Build history of the part. All positions in model axes, mm. A direction names the side the tool comes from. Give positions to 0.01 mm unless a question says otherwise; leave off trailing zeros. Loops run counter-clockwise (first coordinate to the right, second up) from the corner with the lowest first, then second, coordinate; pieces in that order, holes last. Notation, with made-up numbers: M -19,46 L -15,46 A28 ccw -15,69 Z; hole C 15,-31.5 d1. An arc over 180 degrees is marked long. Answer as a JSON object with one key per item and string values. Group by question number.
1. Drill centre lines: line 1 along Y through (x, z) = (35, 3); line 2 along Z through (x, y) = (0, -4.5); line 3 along Z through (x, y) = (-44, -4). Where is each one in solid material? Low to high. Write a range as [from, to].
2. Slice it at C-C (z = 27.5). List the corners of the cut face in (x, y), then the cut area to 3 significant figures.
3. Slice it at A-A (x = -35). List the corners of the cut face in (y, z).
4. Drop flat-ended pins along their axis: pin 1 Ø1.5 at (y, z) = (-15, 49) entering from +X; pin 2 Ø11 at (y, z) = (-7.5, 32.5) entering from -X; pin 3 Ø7 at (y, z) = (-7, 33.5) entering from +X. Give the stop position or say it passes through.
5. 3-axis set-ups, long thin cutter, end or side, ignore diameter. For faces 1 (the face through (-20, -10, 29)), 2 (the face through (-1, 0, 0)), 3 (the face through (0, 0, 33)): which of +Z, -Z, +X, -X, +Y, -Y reach the whole face in a straight line?
6. Slice it at B-B (y = -4). List the corners of the cut face in (x, z), then the cut area to 3 significant figures.
7. Slice it at D-D (z = 8). List the corners of the cut face in (x, y), then the cut area to 3 significant figures.
8. Mould opens along Y. For faces 4 (the face through (-31.38, -19.14, 14.1)), 5 (the face through (-40, 10, 7)), 6 (the face through (1, 20, 6)) say: released by +Y, released by -Y, zero draft, split by the parting line, or undercut.
from build123d import *

# Parameters (mm, degrees)
F0_R     = 5
F0_W     = 40
F0_H     = 40
F1_DEPTH = 15
F2_R     = 5
F3_DEPTH = 20
F4_R     = 3


with BuildPart() as f1:
    # F0 (on Top) → F1 (new body)
    with BuildSketch(Plane.XY):
        with BuildLine():
            Line((-40, -20), (-20.3233100474, -20))
            Line((-20.3233100474, -20), (-20.3233100474, 20))
            Line((-20.3233100474, 20), (-40, 20))
            ThreePointArc((-40, 20), (-47.0710678119, 17.0710678119), (-50, 10))
            Line((-50, 10), (-50, -10))
            ThreePointArc((-50, -10), (-47.0710678119, -17.0710678119), (-40, -20))
        make_face()
        with Locations((-35, 10)):
            Circle(F0_R, mode=Mode.SUBTRACT)
        with Locations((-0.3233100474, 0)):
            Rectangle(F0_W, F0_H)
        with BuildLine():
            Line((19.6766899526, -20), (40, -20))
            ThreePointArc((40, -20), (47.0710678119, -17.0710678119), (50, -10))
            Line((50, -10), (50, 10))
            ThreePointArc((50, 10), (47.0710678119, 17.0710678119), (40, 20))
            Line((40, 20), (19.6766899526, 20))
            Line((19.6766899526, 20), (19.6766899526, -20))
        make_face()
        with Locations((35, 10)):
            Circle(F0_R, mode=Mode.SUBTRACT)
    extrude(amount=F1_DEPTH)

    # F2 (on face) → F3 (join)
    with BuildSketch(Plane.XZ.offset(20)):
        with BuildLine():
            ThreePointArc((20, 40), (0, 60), (-20, 40))
            Line((-20, 40), (-20, 15))
            Line((-20, 15), (20, 15))
            Line((20, 15), (20, 40))
        make_face()
        with Locations((0, 40)):
            Circle(F2_R, mode=Mode.SUBTRACT)
    extrude(amount=-F3_DEPTH)

    # F4
    f4_edges = [f1.edges().sort_by_distance(p)[0] for p in [
        (0, 0, 60),
        (0, 0, 15),
        (0, -20, 60),
        (-30, -20, 15),
        (-20, -20, 27.5),
        (20, -20, 27.5),
        (30, -20, 15),
        (-47.071068, -17.071068, 15),
        (47.071068, -17.071068, 15),
        (-50, 0, 15),
        (-47.071068, 17.071068, 15),
        (0, 20, 15),
        (47.071068, 17.071068, 15),
        (50, 0, 15),
        (20, -10, 15),
        (-20, -10, 15),
        (20, 0, 27.5),
        (-20, 0, 27.5),
    ]]
    fillet(f4_edges, radius=F4_R)


solid = f1.part
Established:
{
 "1": {"line 1": "y = [-20, 5], [15, 20]", "line 2": "z = [0, 35], [45, 60]", "line 3": "z = [0, 15]"},
 "2": {"outline": "M -20,-17 A3 ccw -17,-20 L 17,-20 A3 ccw 20,-17 L 20,-3 A3 ccw 17,0 L -17,0 A3 ccw -20,-3 Z", "area": "792 mm^2"},
 "3": {"outline": "M -20,0 L 5,0 L 5,15 L -17,15 A3 ccw -20,12 Z; M 15,0 L 20,0 L 20,12 A3 ccw 17,15 L 15,15 Z"},
 "4": {"pin 1": "stops at x = 18.22", "pin 2": "stops at x = -20", "pin 3": "stops at x = 20"},
 "5": {"face 1": "+Z, -X, +Y, -Y", "face 2": "-Z, +X, -X, +Y, -Y", "face 3": "+Z, +X, -X, +Y"},
 "6": {"outline": "M -50,0 L 50,0 L 50,12 A3 ccw 47,15 L 23,15 A3 cw 20,18 L 20,40 A20 ccw -20,40 L -20,18 A3 cw -23,15 L -47,15 A3 ccw -50,12 Z; hole C 0,40 d10", "area": "3,050 mm^2"},
 "7": {"outline": "M -50,-10 A10 ccw -40,-20 L 40,-20 A10 ccw 50,-10 L 50,10 A10 ccw 40,20 L -40,20 A10 ccw -50,10 Z; hole C -35,10 d10; hole C 35,10 d10", "area": "3,760 mm^2"},
 "8": {"face 4": "released by -Y", "face 5": "undercut", "face 6": "released by +Y"}
}
